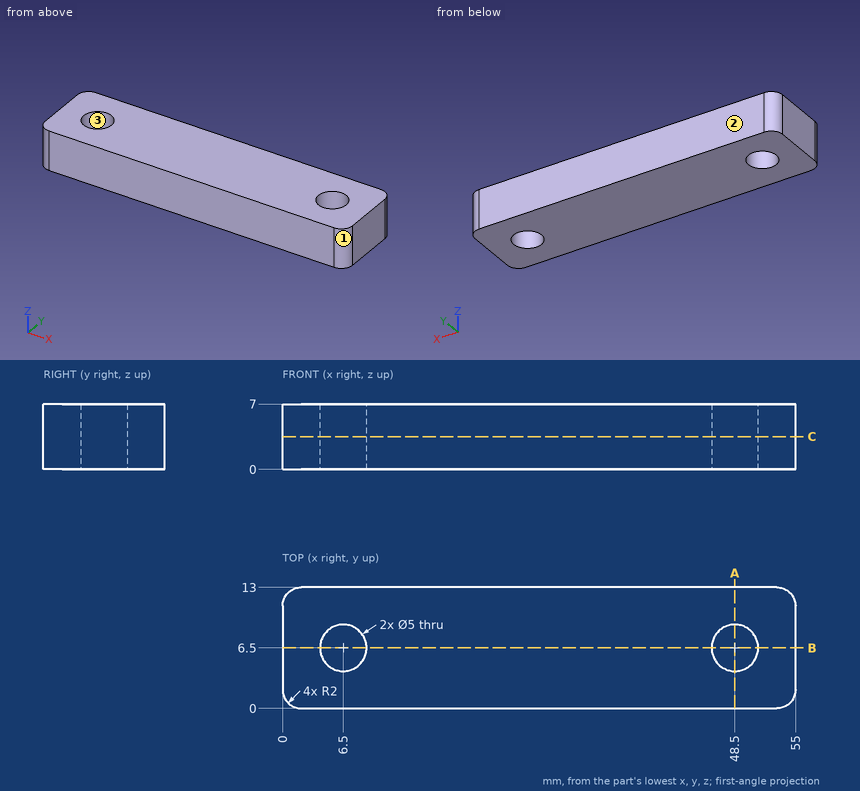
Part print with two shaded views. Sizes in mm from the minimum x, y, z corner. Round coordinates to 2 decimals unless told otherwise and drop trailing zeros. Order: outer loops, then holes, each group sorted by start corner. A loop starts at its lowest first (then second) coordinate and runs counter-clockwise, first axis right, second up. Notation, with made-up numbers: (78, 66.25) -> (93, 66.25) arc R11 cw to (93, 86.25) -> close; hole circle Ø9 at (57, -14.75). An arc over 180 degrees is marked (long way). Use one line per item in the form item = value.
Item 1: Drill centre lines: line 1 (Y direction, x = 48.5, z = 1.5); line 2 (X direction, y = 5, z = 3); line 3 (X direction, y = 8.5, z = 2.75). Where is each one in solid material? Low to high.
Returned:
line_1 = 0 to 4, 9 to 13
line_2 = 0 to 4.5, 8.5 to 46.5, 50.5 to 55
line_3 = 0 to 5, 8 to 47, 50 to 55
Item 2: Cut at B-B, the plane y = 6.5. Write the cut outline in (x, z).
Returned:
outline = (0, 0) -> (4, 0) -> (4, 7) -> (0, 7) -> close; (9, 0) -> (46, 0) -> (46, 7) -> (9, 7) -> close; (51, 0) -> (55, 0) -> (55, 7) -> (51, 7) -> close
Item 3: Cut at C-C, the plane z = 3.5. Write the cut outline in (x, y), and give its area (3 significant figures).
Returned:
outline = (0, 2) arc R2 ccw to (2, 0) -> (53, 0) arc R2 ccw to (55, 2) -> (55, 11) arc R2 ccw to (53, 13) -> (2, 13) arc R2 ccw to (0, 11) -> close; hole circle Ø5 at (6.5, 6.5); hole circle Ø5 at (48.5, 6.5)
area = 672 mm^2
Item 4: Pull direction Y, two halves, no side cores. Call the marked faces 1, 2 and 3: released by +Y, released by -Y, zero draft, split by the parting line, or undercut.
Returned:
face_1 = released by -Y
face_2 = released by +Y
face_3 = undercut
Item 5: Flat gauge pin, fed straight in: pin 1 Ø4 at (x, y) = (6.5, 6.5) entering from -Z. Where does the tip first touch, or does it go through?
Returned:
pin_1 = through
Item 6: Cut at A-A, the plane x = 48.5. Write the cut outline in (y, z), and give its area (3 significant figures).
Returned:
outline = (0, 0) -> (4, 0) -> (4, 7) -> (0, 7) -> close; (9, 0) -> (13, 0) -> (13, 7) -> (9, 7) -> close
area = 56.0 mm^2
